Answer from the drawing. Dimensions are ordinates in mm from the lowest x, y and z of the part. A direction names the side the tool comes from. Give positions to 0.01 mm unless a question says otherwise; leave off trailing zeros. Write each loop counter-clockwise with the first axis right and the second up, starting at its lowest first coordinate (ties: lowest second). Pieces come first, ordered by that corner, then holes. Notation, with made-up numbers: (-4.75, -21.5) -> (19.25, -21.5) arc R24 ccw to (19.25, -0.5) -> close; hole circle Ø10 at (86, 23.5). An arc over 180 degrees is marked (long way). Use a Markdown table: item, result. Add a question column.
Q1. For a pull along Z with two mould halves and no side action, classify the marked faces 4, 5 and 6 as pulls with the +Z half, pulls with the -Z half, needs draft (parallel to the pull), parting line crosses it, or undercut.
Q2. Consider line 1 (X direction, y = 27, z = 12) (1 decimal); line 2 (X direction, y = 83.5, z = 17) (1 decimal); line 3 (Y direction, x = 127, z = 64). Determine where each line is inside the solid, lowest interval first.
Q3. Section A-A, the plane z = 58 is taken. Give the vertices of the cut face in (x, y) (1 decimal), plus the area to 3 significant figures.
Q4. For the marked faces 1, 2 and 3, determine the directions among +Z, -Z, +X, -X, +Y, -Y from which every point of the face is accessible in a straight line to the end or side of a thin tool.
Q5. Section B-B, the plane z = 172 is taken. Give the vertices of the cut face in (x, y) (1 decimal), plus the area to 3 significant figures.
Q6. Each of these flat-tipped pins is pushed along its axis until it touches: pin 1 Ø13 at (x, z) = (15.5, 50) entering from -Y; pin 2 Ø22 at (y, z) = (99, 7.5) entering from +X; pin 3 Ø10 at (y, z) = (43, 5) entering from -X. Where does it stop, or does it pass through?
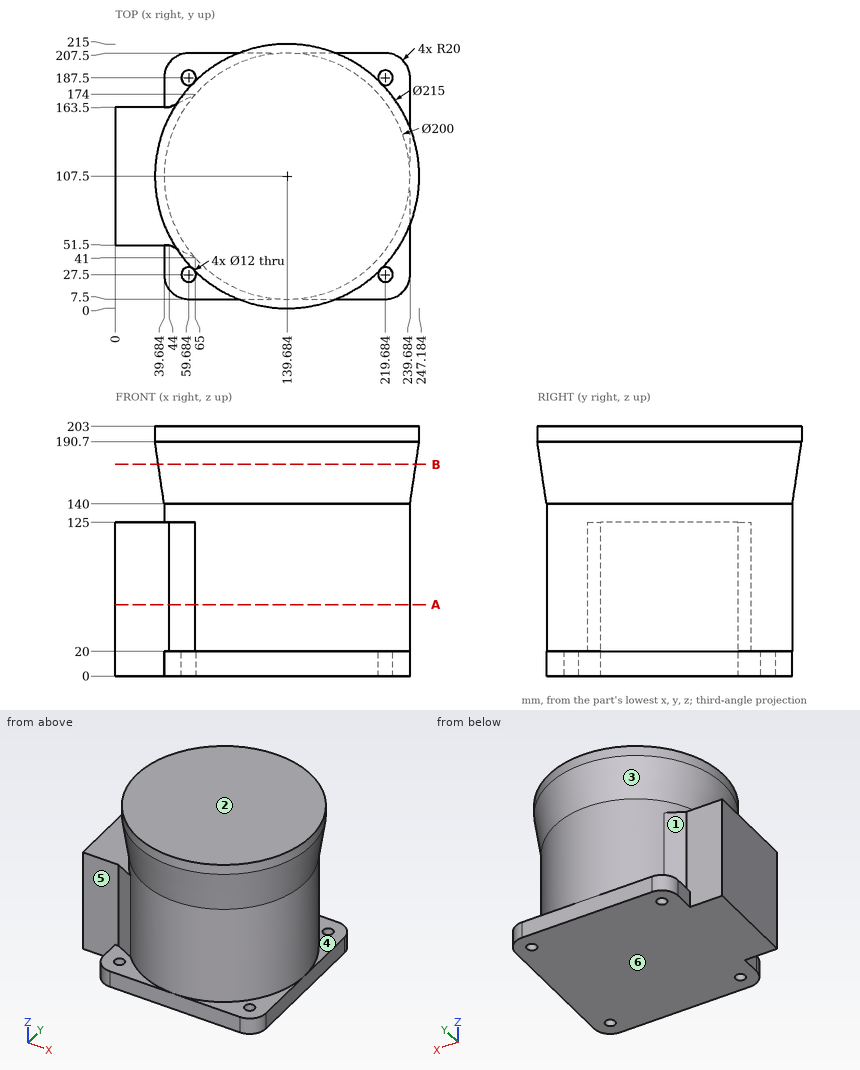
Result set:
| question | item | result |
|---|---|---|
| 1 | face 4 | undercut |
| 1 | face 5 | needs draft |
| 1 | face 6 | pulls with the -Z half |
| 2 | line 1 | x = 39.7 to 53.7, 65.7 to 213.7, 225.7 to 239.7 |
| 2 | line 2 | x = 0 to 239.7 |
| 2 | line 3 | y = 8.31 to 206.69 |
| 3 | outline | (0, 51.5) -> (44, 51.5) -> (65, 41) arc R100 ccw (long way) to (65, 174) -> (44, 163.5) -> (0, 163.5) -> close |
| 3 | area | 36,600 mm2 |
| 4 | face 1 | -X, +Y |
| 4 | face 2 | +Z, +X, -X, +Y, -Y |
| 4 | face 3 | none |
| 5 | outline | circle Ø209.5 at (139.7, 107.5) |
| 5 | area | 34,500 mm2 |
| 6 | pin 1 | stops at y = 51.5 |
| 6 | pin 2 | stops at x = 239.68 |
| 6 | pin 3 | stops at x = 39.68 |
